from build123d import *

# Parameters (mm, degrees)
SKETCH1_W               = 290
SKETCH1_H               = 290
BOSS_EXTRUDE1_DEPTH     = 47
SKETCH2_R               = 65.5
CUT_EXTRUDE1_DEPTH      = 40
SKETCH3_R               = 80.5
CUT_EXTRUDE2_DEPTH      = 1
SKETCH4_OUTSIDE_W       = 374.562
SKETCH4_OUTSIDE_H       = 374.562
SKETCH4_OUTSIDE_R       = 74.125
CUT_EXTRUDE3_DEPTH      = 21.33
CUT_EXTRUDE4_DEPTH      = 413.806249953
CUT_EXTRUDE4_DEPTH_BACK = 413.806249953
SKETCH5_R               = 34
CUT_EXTRUDE5_DEPTH      = 413.806249953
CUT_EXTRUDE5_DEPTH_BACK = 413.806249953
SKETCH6_R               = 7.65
SKETCH7_R               = 80.5
SKETCH7_R_2             = 74.125
CUT_EXTRUDE6_DEPTH      = 15
SKETCH8_W               = 4
SKETCH8_H               = 55
CUT_EXTRUDE7_DEPTH      = 2
CUT_EXTRUDE8_DEPTH      = 411.92450511
CUT_EXTRUDE8_DEPTH_BACK = 411.92450511
SKETCH9_OUTSIDE_W       = 374.562
SKETCH9_OUTSIDE_H       = 374.562
SKETCH9_OUTSIDE_R       = 144


with BuildPart() as part:
    # Sketch1 → Boss-Extrude1 (new body)
    with BuildSketch(Plane(origin=(0, 0, 0), x_dir=(1, 0, 0), z_dir=(0, 1, 0))):
        with Locations((145, -145)):
            Rectangle(SKETCH1_W, SKETCH1_H)
    extrude(amount=BOSS_EXTRUDE1_DEPTH)

    # Sketch2 → Cut-Extrude1 (cut)
    with BuildSketch(Plane(origin=(0, 47, 0), x_dir=(1, 0, 0), z_dir=(0, 1, 0))):
        with Locations(Location((145, -145, 0), (0, 0, 270))):
            Circle(SKETCH2_R)
    extrude(amount=-CUT_EXTRUDE1_DEPTH, mode=Mode.SUBTRACT)

    # Sketch3 → Cut-Extrude2 (cut)
    with BuildSketch(Plane(origin=(0, 47, 0), x_dir=(1, 0, 0), z_dir=(0, 1, 0))):
        with Locations(Location((145, -145, 0), (0, 0, 270))):
            Circle(SKETCH3_R)
    extrude(amount=-CUT_EXTRUDE2_DEPTH, mode=Mode.SUBTRACT)

    # Sketch4 outside → Cut-Extrude3 (cut)
    with BuildSketch(Plane.XZ):
        with Locations((145, 145)):
            Rectangle(SKETCH4_OUTSIDE_W, SKETCH4_OUTSIDE_H)
        with Locations(Location((145, 145, 0), (0, 0, 270))):
            Circle(SKETCH4_OUTSIDE_R, mode=Mode.SUBTRACT)
    extrude(amount=-CUT_EXTRUDE3_DEPTH, mode=Mode.SUBTRACT)

    # Sketch5 → Cut-Extrude4 (cut, two sides: drawn at the far end of the back side and taken through both)
    with BuildSketch(Plane.XZ.offset(-CUT_EXTRUDE4_DEPTH_BACK)):
        with Locations(Location((145, 145, 0), (0, 0, 90))):
            Circle(SKETCH5_R)
    extrude(amount=CUT_EXTRUDE4_DEPTH + CUT_EXTRUDE4_DEPTH_BACK, mode=Mode.SUBTRACT)

    # Sketch6 → Cut-Extrude5 (cut, two sides: drawn at the far end of the back side and taken through both)
    with BuildSketch(Plane.XZ.offset(-CUT_EXTRUDE5_DEPTH_BACK)):
        with Locations(Location((145, 200, 0), (0, 0, 90))):
            Circle(SKETCH6_R)
        with Locations(Location((197.308108396, 161.995934691, 0), (0, 0, 90))):
            Circle(SKETCH6_R)
        with Locations(Location((177.328188876, 100.504065309, 0), (0, 0, 90))):
            Circle(SKETCH6_R)
        with Locations(Location((112.671811124, 100.504065309, 0), (0, 0, 90))):
            Circle(SKETCH6_R)
        with Locations(Location((92.691891604, 161.995934691, 0), (0, 0, 90))):
            Circle(SKETCH6_R)
    extrude(amount=CUT_EXTRUDE5_DEPTH + CUT_EXTRUDE5_DEPTH_BACK, mode=Mode.SUBTRACT)

    # Sketch7 → Cut-Extrude6 (cut)
    with BuildSketch(Plane.XZ.offset(-21.33)):
        with Locations(Location((145, 145, 0), (0, 0, 90))):
            Circle(SKETCH7_R)
        with Locations(Location((145, 145, 0), (0, 0, 270))):
            Circle(SKETCH7_R_2, mode=Mode.SUBTRACT)
    extrude(amount=-CUT_EXTRUDE6_DEPTH, mode=Mode.SUBTRACT)

    # Sketch8 → Cut-Extrude7 (cut)
    with BuildSketch(Plane.XZ.offset(-21.33)):
        Polygon((254.921555667, 230.101419493), (211.920824131, 195.809480391), (209.426864924, 198.936806321), (252.427596459, 233.228745423), align=None)
        with Locations((145, 256.5)):
            Rectangle(SKETCH8_W, SKETCH8_H)
        Polygon((280.069937925, 112.119734356), (226.448902755, 124.358385723), (227.338986491, 128.258097372), (280.960021661, 116.019446004), align=None)
        Polygon((203.507902002, 18.897559883), (179.64429635, 68.450847618), (183.248171822, 70.186382574), (207.111777473, 20.63309484), align=None)
        Polygon((82.888222527, 20.63309484), (106.751828178, 70.186382574), (110.35570365, 68.450847618), (86.492097998, 18.897559883), align=None)
        Polygon((9.039978339, 116.019446004), (62.661013509, 128.258097372), (63.551097245, 124.358385723), (9.930062075, 112.119734356), align=None)
        Polygon((37.572403541, 233.228745423), (80.573135076, 198.936806321), (78.079175869, 195.809480391), (35.078444333, 230.101419493), align=None)
    extrude(amount=-CUT_EXTRUDE7_DEPTH, mode=Mode.SUBTRACT)

    # Sketch9 outside → Cut-Extrude8 (cut, two sides: drawn at the far end of the back side and taken through both)
    with BuildSketch(Plane.XZ.offset(-21.33).offset(-CUT_EXTRUDE8_DEPTH_BACK)):
        with Locations((145, 145)):
            Rectangle(SKETCH9_OUTSIDE_W, SKETCH9_OUTSIDE_H)
        with Locations(Location((145, 145, 0), (0, 0, 270))):
            Circle(SKETCH9_OUTSIDE_R, mode=Mode.SUBTRACT)
    extrude(amount=CUT_EXTRUDE8_DEPTH + CUT_EXTRUDE8_DEPTH_BACK, mode=Mode.SUBTRACT)


solid = part.part
Geometry check sheet. Reference: the model listing, model coordinates, mm. A direction names the side the tool comes from. Round coordinates to 2 decimals unless told otherwise and drop trailing zeros. Loops run counter-clockwise (first coordinate to the right, second up) from the corner with the lowest first, then second, coordinate; pieces in that order, holes last.
Item 1: Gauge pin test, flat ends, axial feed: pin 1 (5 mm diameter, centred on x = 216, y = 23.5, fed in from -Z); pin 2 (1 mm diameter, centred on x = 236, z = 145.5, fed in from -Y); pin 3 (2 mm diameter, centred on y = 22.5, z = 250.5, fed in from +X). Record the tip position at first contact, or that the pin passes through.
Item 2: Access from +Z, -Z, +X, -X, +Y, -Y to the whole of each face (thin tool, end or side, straight path). Record for faces 1 (the flat face through (37.116, 22.316, 118.325)), 2 (the cylindrical face through (224.815, 46.507, 134.521)), 3 (the cylindrical face through (178.19, 3.55, 137.63)).
Item 3: Cross-section at D-D on z = 102. Record the boundary of the cut face in (x, y), then the cut area to 3 significant figures.
Item 4: Thickness scan on line 1 (X direction, y = 34, z = 145) (3 decimals); line 2 (Z direction, x = 139, y = 6); line 3 (Y direction, x = 109.5, z = 131.5). Record the ranges inside material, lowest first.
Item 5: Mould release check, pull along X, two halves, no side actions. Record for faces 4 (the flat face through (233.722, 22.316, 213.195)), 5 (the flat face through (207, 21.33, 83)), 6 (the cylindrical face through (4.424, 34.345, 176.216)): pulls with the +X half, pulls with the -X half, needs draft (parallel to the pull), parting line crosses it, or undercut.
Item 6: Cross-section at B-B on y = 12.5. Record the boundary of the cut face in (x, z) (3 decimals).
Item 7: Cross-section at C-C on x = 265.5. Record the boundary of the cut face in (y, z), then the cut area to 3 significant figures.
Item 8: Cross-section at A-A on z = 145. Record the boundary of the cut face in (x, y) (3 decimals).
Answer sheet:
1. pin 1: stops at z = 18.34
1. pin 2: stops at y = 21.33
1. pin 3: stops at x = 244.07
2. face 1: -Y
2. face 2: +Y
2. face 3: +Y, -Y
3. outline: (7.57, 21.33) - (76.95, 21.33) - (76.95, 36.33) - (84.62, 36.33) - (84.62, 0) - (105.17, 0) - (105.17, 7) - (95.59, 7) - (95.59, 46) - (76.95, 46) - (76.95, 47) - (7.57, 47) - close; (120.17, 0) - (169.83, 0) - (169.83, 7) - (120.17, 7) - close; (184.83, 0) - (205.38, 0) - (205.38, 36.33) - (213.05, 36.33) - (213.05, 21.33) - (282.43, 21.33) - (282.43, 47) - (213.05, 47) - (213.05, 46) - (194.41, 46) - (194.41, 7) - (184.83, 7) - close
3. area: 5,200 mm2
4. line 1: x = 1 to 64.5, 70.875 to 79.5, 210.5 to 219.125, 225.5 to 289
4. line 2: z = 71.12 to 111.53, 178.47 to 195.25, 204.75 to 218.88
4. line 3: y = 0 to 7
5. face 4: undercut
5. face 5: needs draft
5. face 6: parting line crosses it
6. outline: circle Ø148.25 at (145, 145); hole circle Ø131 at (145, 145)
7. outline: (21.33, 66.16) - (47, 66.16) - (47, 223.84) - (21.33, 223.84) - (21.33, 119.55) - (23.33, 119.55) - (23.33, 115.45) - (21.33, 115.45) - close
7. area: 4,040 mm2
8. outline: (1, 21.33) - (64.5, 21.33) - (64.5, 36.33) - (70.875, 36.33) - (70.875, 0) - (111, 0) - (111, 7) - (79.5, 7) - (79.5, 46) - (64.5, 46) - (64.5, 47) - (1, 47) - close; (179, 0) - (219.125, 0) - (219.125, 36.33) - (225.5, 36.33) - (225.5, 21.33) - (289, 21.33) - (289, 47) - (225.5, 47) - (225.5, 46) - (210.5, 46) - (210.5, 7) - (179, 7) - close
